Check sheet for the modelled part. Datum: model origin and axes. Units: mm. A direction names the side the tool comes from. Round coordinates to 2 decimals unless told otherwise and drop trailing zeros. Loops run counter-clockwise (first coordinate to the right, second up) from the corner with the lowest first, then second, coordinate; pieces in that order, holes last. Notation, with made-up numbers: M 29.25,27 L 75.25,27 A6 ccw 75.25,31 Z; hole C -32.75,61.5 d2. An arc over 180 degrees is marked long. Write item = value, one per line. Start each with the question number.
(1) Go/stop test with a flat-tipped pin: P1, Ø1.2, axis at x = 1, y = 2.5, coming from the +Z side. Record where the tip stops, or that it passes through.
(2) Cross-section at A-A on x = 38.95. Record the boundary of the cut face in (y, z).
(3) Cross-section at C-C on z = 25. Record the boundary of the cut face in (x, y).
(4) Cross-section at B-B on y = 25.5. Record the boundary of the cut face in (x, z).
(5) Scan lines: L1, parallel to Z at x = 38.95, y = -1; L2, parallel to Y at x = 33.5, z = 12.5. Record each from-to range of solid material in increasing order. Write a range as from..to.
(6) Mould release check, pull along X, two halves, no side actions. Record for faces 4 (the face through (22.9, -0.4, 51.5)), 5 (the face through (20, 51, 46.569)), 6 (the face through (-1.5, 25, 26)): pulls with the +X half, pulls with the -X half, needs draft (parallel to the pull), parting line crosses it, or undercut.
(7) Set-up check for faces 1 (the face through (1, 46, 43.85)), 2 (the face through (46.569, 51, 21)), 3 (the face through (1, 4, 48.22)): record each of +Z, -Z, +X, -X, +Y, -Y from which the full face is reachable in a straight line by a thin tool's end or side.
(8) Cross-section at D-D on y = 2.5. Record the boundary of the cut face in (x, z), plus the area to 3 significant figures.
from build123d import *

# Parameters (mm, degrees)
SKETCH1_W                      = 53
SKETCH1_H                      = 53
BOSS_EXTRUDE1_DEPTH            = 51.5
SKETCH2_W                      = 50
SKETCH2_H                      = 50
CUT_EXTRUDE1_DEPTH             = 50
SKETCH3_W                      = 1.5
SKETCH3_H                      = 1.5
CUT_EXTRUDE2_DEPTH             = 90.20061659
SKETCH4_W                      = 1.5
SKETCH4_H                      = 1.5
CUT_EXTRUDE3_DEPTH             = 90.20061659
SKETCH5_W                      = 1.5
SKETCH5_H                      = 1.5
CUT_EXTRUDE4_DEPTH             = 90.20061659
SKETCH6_W                      = 1.5
SKETCH6_H                      = 1.5
CUT_EXTRUDE5_DEPTH             = 90.20061659
SKETCH7_W                      = 1.5
SKETCH7_H                      = 1.5
CUT_EXTRUDE6_DEPTH             = 90.20061659
CUT_EXTRUDE7_REACH             = 92.075
SKETCH8_W                      = 1.5
SKETCH8_H                      = 1.5
F_16_0_16_DIAMETER_HOLE1_D     = 16
F_16_0_16_DIAMETER_HOLE1_DEPTH = 1.5
F_2_3_2_3_DIAMETER_HOLE1_D     = 2.3
F_2_3_2_3_DIAMETER_HOLE1_DEPTH = 1.5
F_16_0_16_DIAMETER_HOLE2_D     = 16
F_16_0_16_DIAMETER_HOLE2_DEPTH = 1.5
RIB1_START                     = -2.185
RIB1_OUTLINE_W                 = 1.5
RIB1_OUTLINE_H                 = 8
RIB1_DEPTH                     = 4.37
RIB2_START                     = -2.185
RIB2_OUTLINE_W                 = 1.5
RIB2_OUTLINE_H                 = 8
RIB2_DEPTH                     = 4.37
RIB3_START                     = -2.185
RIB3_OUTLINE_W                 = 1.5
RIB3_OUTLINE_H                 = 8
RIB3_DEPTH                     = 4.37
RIB4_START                     = -2.185
RIB4_OUTLINE_W                 = 1.5
RIB4_OUTLINE_H                 = 8
RIB4_DEPTH                     = 4.37


# Read off the part's stored shape, not the designer's step: Rib1, Rib2, Rib3, Rib4
with BuildPart() as part:
    # Sketch1 → Boss-Extrude1 (new body)
    with BuildSketch(Plane.XY.offset(51.5)):
        with Locations((25, 25)):
            Rectangle(SKETCH1_W, SKETCH1_H)
    extrude(amount=-BOSS_EXTRUDE1_DEPTH)

    # Sketch2 → Cut-Extrude1 (cut)
    with BuildSketch(Plane.XY.offset(51.5)):
        with Locations((25, 25)):
            Rectangle(SKETCH2_W, SKETCH2_H)
    extrude(amount=-CUT_EXTRUDE1_DEPTH, mode=Mode.SUBTRACT)

    # Sketch3 → Cut-Extrude2 (cut, through all)
    with BuildSketch(Plane.XZ.offset(-50)):
        with Locations((45.818516526, 21.323619098)):
            Rectangle(SKETCH3_W, SKETCH3_H)
    extrude(amount=-CUT_EXTRUDE2_DEPTH, mode=Mode.SUBTRACT)

    # Sketch4 → Cut-Extrude3 (cut, through all)
    with BuildSketch(Plane.XZ.offset(-50)):
        with Locations((10.857864376, 13.857864376)):
            Rectangle(SKETCH4_W, SKETCH4_H)
    extrude(amount=-CUT_EXTRUDE3_DEPTH, mode=Mode.SUBTRACT)

    # Sketch5 → Cut-Extrude4 (cut, through all)
    with BuildSketch(Plane.XZ.offset(-50)):
        with Locations((19.823619098, 47.318516526)):
            Rectangle(SKETCH5_W, SKETCH5_H)
    extrude(amount=-CUT_EXTRUDE4_DEPTH, mode=Mode.SUBTRACT)

    # Sketch6 → Cut-Extrude5 (cut, through all)
    with BuildSketch(Plane.XZ.offset(-50)):
        with Locations((19.823619098, 44.318516526)):
            Rectangle(SKETCH6_W, SKETCH6_H)
    extrude(amount=-CUT_EXTRUDE5_DEPTH, mode=Mode.SUBTRACT)

    # Sketch7 → Cut-Extrude6 (cut, through all)
    with BuildSketch(Plane.XZ.offset(-50)):
        with Locations((10.857864376, 10.857864376)):
            Rectangle(SKETCH7_W, SKETCH7_H)
    extrude(amount=-CUT_EXTRUDE6_DEPTH, mode=Mode.SUBTRACT)

    # Sketch8 → Cut-Extrude7 (cut, up to next)
    with BuildSketch(Plane(origin=(0, 51.5, 0), x_dir=(-1, 0, 0), z_dir=(0, 1, 0)), mode=Mode.PRIVATE) as cut_extrude7_sk1:
        with Locations((-42.818516526, 21.323619098)):
            Rectangle(SKETCH8_W, SKETCH8_H)
    cut_extrude7_tool1 = extrude(cut_extrude7_sk1.sketch, amount=-CUT_EXTRUDE7_REACH, mode=Mode.PRIVATE) & part.part
    add(cut_extrude7_tool1.solids().sort_by_distance((42.818517, 51.5, 21.323619))[0], mode=Mode.SUBTRACT)

    # Ø16.0 (16) Diameter Hole1
    with Locations(Plane(origin=(0, -1.5, 0), x_dir=(-1, 0, 0), z_dir=(0, -1, 0))):
        with Locations((-25, -25)):
            Hole(F_16_0_16_DIAMETER_HOLE1_D / 2, depth=F_16_0_16_DIAMETER_HOLE1_DEPTH)

    # Ø2.3 (2.3) Diameter Hole1
    with Locations(Plane(origin=(0, 0, 0), x_dir=(1, 0, 0), z_dir=(0, 1, 0))):
        with Locations((38.95, -11.05), (11.05, -11.05), (11.05, -38.95), (38.95, -38.95)):
            Hole(F_2_3_2_3_DIAMETER_HOLE1_D / 2, depth=F_2_3_2_3_DIAMETER_HOLE1_DEPTH)

    # Ø16.0 (16) Diameter Hole2
    with Locations(Plane(origin=(0, 51.5, 0), x_dir=(1, 0, 0), z_dir=(0, 1, 0))):
        with Locations((25, -26.5)):
            Hole(F_16_0_16_DIAMETER_HOLE2_D / 2, depth=F_16_0_16_DIAMETER_HOLE2_DEPTH)

    # Rib1 outline → Rib1 (add)
    with BuildSketch(Plane(origin=(0, 0, 46.035), x_dir=(-1, 0, 0), z_dir=(0, 0, -1)).offset(RIB1_START)):
        with Locations((-49.25, 46)):
            Rectangle(RIB1_OUTLINE_W, RIB1_OUTLINE_H)
    extrude(amount=RIB1_DEPTH)

    # Rib2 outline → Rib2 (add)
    with BuildSketch(Plane(origin=(0, 0, 46.035), x_dir=(-1, 0, 0), z_dir=(0, 0, -1)).offset(RIB2_START)):
        with Locations((-0.75, 4)):
            Rectangle(RIB2_OUTLINE_W, RIB2_OUTLINE_H)
    extrude(amount=RIB2_DEPTH)

    # Rib3 outline → Rib3 (add)
    with BuildSketch(Plane.XY.offset(46.035).offset(RIB3_START)):
        with Locations((0.75, 46)):
            Rectangle(RIB3_OUTLINE_W, RIB3_OUTLINE_H)
    extrude(amount=RIB3_DEPTH)

    # Rib4 outline → Rib4 (add)
    with BuildSketch(Plane.XY.offset(46.035).offset(RIB4_START)):
        with Locations((49.25, 4)):
            Rectangle(RIB4_OUTLINE_W, RIB4_OUTLINE_H)
    extrude(amount=RIB4_DEPTH)


solid = part.part
Result:
q1.P1 = 48.22
q2.outline = M -1.5,0 L 51.5,0 L 51.5,51.5 L 50,51.5 L 50,1.5 L 0,1.5 L 0,9.9 L -1.5,9.9 Z; M -1.5,12.2 L 0,12.2 L 0,37.8 L -1.5,37.8 Z; M -1.5,40.1 L 0,40.1 L 0,51.5 L -1.5,51.5 Z
q3.outline = M -1.5,-1.5 L 17,-1.5 L 17,0 L 0,0 L 0,50 L 17.14,50 L 17.14,51.5 L -1.5,51.5 Z; M 32.86,50 L 50,50 L 50,0 L 33,0 L 33,-1.5 L 51.5,-1.5 L 51.5,51.5 L 32.86,51.5 Z
q4.outline = M -1.5,0 L 51.5,0 L 51.5,51.5 L 50,51.5 L 50,1.5 L 0,1.5 L 0,51.5 L -1.5,51.5 Z
q5.L1 = 0..9.9, 12.2..37.8, 40.1..51.5
q5.L2 = -1.5..0, 50..51.5
q6.face_4 = needs draft
q6.face_5 = undercut
q6.face_6 = pulls with the -X half
q7.face_1 = none
q7.face_2 = +Y
q7.face_3 = +Z
q8.outline = M -1.5,0 L 51.5,0 L 51.5,51.5 L 50,51.5 L 50,48.22 L 48.5,48.22 L 48.5,43.85 L 50,43.85 L 50,1.5 L 0,1.5 L 0,43.85 L 1.5,43.85 L 1.5,48.22 L 0,48.22 L 0,51.5 L -1.5,51.5 Z
q8.area = 243 mm^2
